Build history of the part. All positions in model axes, mm. A direction names the side the tool comes from. Round coordinates to 2 decimals unless told otherwise and drop trailing zeros. Write each loop counter-clockwise with the first axis right and the second up, starting at its lowest first coordinate (ties: lowest second). Pieces come first, ordered by that corner, then holes. Notation, with made-up numbers: M 9,79 L 37,79 A16 cw 37,110 Z; hole C 44.5,77 d9. An arc over 180 degrees is marked long. Write item = value, one per line.
Autodesk Fusion 360 part; units mm, degrees
sketch "Sketch1" plane through (0, 0, 0) normal (0, 1, 0) x (1, 0, 0)
  line L0 (0, 0) -> (88, 0)
  line L1 (88, 0) -> (88, 8.2)
  line L2 (88, 8.2) -> (0, 8.2)
  line L3 (0, 8.2) -> (0, 0)
  dimension "d1" = 88
  dimension "d2" = 8.2
extrude "Extrude1" add sketch "Sketch1" along normal blind 12.75
sketch "Sketch2" plane through (0, 12.75, 0) normal (0, 1, 0) x (-1, 0, 0)
  line L0 (0, -8.2) -> (0, 0)
  line L1 (0, 0) -> (-88, 0)
  line L2 (-88, 0) -> (-88, -8.2)
  line L3 (-88, -8.2) -> (0, -8.2)
  line L4 (0, 0) -> (-6.77, 0)
  line L5 (-6.77, 0) -> (-6.77, -8.2)
  line L6 (-6.77, -8.2) -> (0, -8.2)
  line L7 (0, -8.2) -> (0, 0)
  line L8 (-6.77, -8.2) -> (-13.54, -8.2)
  line L9 (-13.54, -8.2) -> (-13.54, 0)
  line L10 (-13.54, 0) -> (-6.77, 0)
  line L11 (-6.77, 0) -> (-6.77, -8.2)
  dimension "d5" = 6.77
  dimension "d6" = 6.77
extrude "Extrude2" cut sketch "Sketch2" against normal blind 6.5 contours L1 L3 L5 L8 L9 L10 L11
sketch "Sketch3" plane through (0, 12.75, 0) normal (0, 1, 0) x (-1, 0, 0)
  line L0 (-13.54, -8.2) -> (-13.54, 0)
  line L1 (-13.54, 0) -> (-88, 0)
  line L2 (-88, 0) -> (-88, -8.2)
  line L3 (-88, -8.2) -> (-13.54, -8.2)
  line L4 (-13.54, 0) -> (-20.31, 0)
  line L5 (-20.31, 0) -> (-20.31, -8.2)
  line L6 (-20.31, -8.2) -> (-13.54, -8.2)
  line L7 (-13.54, -8.2) -> (-13.54, 0)
  line L8 (-20.31, -8.2) -> (-27.08, -8.2)
  line L9 (-27.08, -8.2) -> (-27.08, 0)
  line L10 (-27.08, 0) -> (-20.31, 0)
  line L11 (-20.31, 0) -> (-20.31, -8.2)
  dimension "d9" = 6.77
  dimension "d10" = 6.77
extrude "Extrude3" cut sketch "Sketch3" against normal blind 6.5 contours L1 L3 L5 L8 L9 L10 L11
sketch "Sketch4" plane through (0, 12.75, 0) normal (0, 1, 0) x (-1, 0, 0)
  line L0 (-27.08, -8.2) -> (-27.08, 0)
  line L1 (-27.08, 0) -> (-88, 0)
  line L2 (-88, 0) -> (-88, -8.2)
  line L3 (-88, -8.2) -> (-27.08, -8.2)
  line L4 (-27.08, 0) -> (-33.85, 0)
  line L5 (-33.85, 0) -> (-33.85, -8.2)
  line L6 (-33.85, -8.2) -> (-27.08, -8.2)
  line L7 (-27.08, -8.2) -> (-27.08, 0)
  line L8 (-33.85, -8.2) -> (-40.62, -8.2)
  line L9 (-40.62, -8.2) -> (-40.62, 0)
  line L10 (-40.62, 0) -> (-33.85, 0)
  line L11 (-33.85, 0) -> (-33.85, -8.2)
  dimension "d13" = 6.77
  dimension "d14" = 6.77
extrude "Extrude4" cut sketch "Sketch4" against normal blind 6.5 contours L1 L3 L5 L8 L9 L10 L11
sketch "Sketch5" plane through (0, 12.75, 0) normal (0, 1, 0) x (-1, 0, 0)
  line L0 (-40.62, -8.2) -> (-40.62, 0)
  line L1 (-40.62, 0) -> (-88, 0)
  line L2 (-88, 0) -> (-88, -8.2)
  line L3 (-88, -8.2) -> (-40.62, -8.2)
  line L4 (-40.62, 0) -> (-47.39, 0)
  line L5 (-47.39, 0) -> (-47.39, -8.2)
  line L6 (-47.39, -8.2) -> (-40.62, -8.2)
  line L7 (-40.62, -8.2) -> (-40.62, 0)
  line L8 (-47.39, -8.2) -> (-54.16, -8.2)
  line L9 (-54.16, -8.2) -> (-54.16, 0)
  line L10 (-54.16, 0) -> (-47.39, 0)
  line L11 (-47.39, 0) -> (-47.39, -8.2)
  dimension "d17" = 6.77
  dimension "d18" = 6.77
extrude "Extrude5" cut sketch "Sketch5" against normal blind 6.5 contours L1 L3 L5 L8 L9 L10 L11
sketch "Sketch6" plane through (0, 12.75, 0) normal (0, 1, 0) x (-1, 0, 0)
  line L0 (-54.16, -8.2) -> (-54.16, 0)
  line L1 (-54.16, 0) -> (-88, 0)
  line L2 (-88, 0) -> (-88, -8.2)
  line L3 (-88, -8.2) -> (-54.16, -8.2)
  line L4 (-54.16, 0) -> (-60.93, 0)
  line L5 (-60.93, 0) -> (-60.93, -8.2)
  line L6 (-60.93, -8.2) -> (-54.16, -8.2)
  line L7 (-54.16, -8.2) -> (-54.16, 0)
  line L8 (-60.93, 0) -> (-67.7, 0)
  line L9 (-67.7, 0) -> (-67.7, -8.2)
  line L10 (-67.7, -8.2) -> (-60.93, -8.2)
  line L11 (-60.93, -8.2) -> (-60.93, 0)
  dimension "d21" = 6.77
  dimension "d22" = 6.77
extrude "Extrude6" cut sketch "Sketch6" against normal blind 6.5 contours L1 L3 L5 L8 L9 L10 L11
sketch "Sketch7" plane through (0, 12.75, 0) normal (0, 1, 0) x (-1, 0, 0)
  line L0 (-67.7, -8.2) -> (-67.7, 0)
  line L1 (-67.7, 0) -> (-88, 0)
  line L2 (-88, 0) -> (-88, -8.2)
  line L3 (-88, -8.2) -> (-67.7, -8.2)
  line L4 (-67.7, 0) -> (-74.47, 0)
  line L5 (-74.47, 0) -> (-74.47, -8.2)
  line L6 (-74.47, -8.2) -> (-67.7, -8.2)
  line L7 (-67.7, -8.2) -> (-67.7, 0)
  line L8 (-74.47, -8.2) -> (-81.24, -8.2)
  line L9 (-81.24, -8.2) -> (-81.24, 0)
  line L10 (-81.24, 0) -> (-74.47, 0)
  line L11 (-74.47, 0) -> (-74.47, -8.2)
  dimension "d25" = 6.77
  dimension "d26" = 6.77
extrude "Extrude7" cut sketch "Sketch7" against normal blind 6.5 contours L1 L3 L5 L8 L9 L10 L11
1. Flat gauge pin, fed straight in: pin 1 (3.5 mm diameter, centred on x = 51, z = -5, fed in from +Y). Where does the tip first touch, or does it go through?
Responses:
pin_1 = 6.25
2. Mould opens along X. For faces 3 (the face through (0, 6, -4)), 4 (the face through (85, 12.75, -4)), 5 (the face through (60.93, 10, -4)) say: pulls with the +X half, pulls with the -X half, needs draft (parallel to the pull), parting line crosses it, or undercut.
Responses:
face_3 = pulls with the -X half
face_4 = needs draft
face_5 = undercut
3. Band-saw the part on B-B (z = -7.25). List the corners of the cut face in (x, y).
Responses:
outline = M 0,0 L 88,0 L 88,12.75 L 81.24,12.75 L 81.24,6.25 L 74.47,6.25 L 74.47,12.75 L 67.7,12.75 L 67.7,6.25 L 60.93,6.25 L 60.93,12.75 L 54.16,12.75 L 54.16,6.25 L 47.39,6.25 L 47.39,12.75 L 40.62,12.75 L 40.62,6.25 L 33.85,6.25 L 33.85,12.75 L 27.08,12.75 L 27.08,6.25 L 20.31,6.25 L 20.31,12.75 L 13.54,12.75 L 13.54,6.25 L 6.77,6.25 L 6.77,12.75 L 0,12.75 Z
4. Band-saw the part on A-A (y = 10). List the corners of the cut face in (x, z), plus the area to 3 significant figures.
Responses:
outline = M 0,-8.2 L 6.77,-8.2 L 6.77,0 L 0,0 Z; M 13.54,-8.2 L 20.31,-8.2 L 20.31,0 L 13.54,0 Z; M 27.08,-8.2 L 33.85,-8.2 L 33.85,0 L 27.08,0 Z; M 40.62,-8.2 L 47.39,-8.2 L 47.39,0 L 40.62,0 Z; M 54.16,-8.2 L 60.93,-8.2 L 60.93,0 L 54.16,0 Z; M 67.7,-8.2 L 74.47,-8.2 L 74.47,0 L 67.7,0 Z; M 81.24,-8.2 L 88,-8.2 L 88,0 L 81.24,0 Z
area = 389 mm²
5. Band-saw the part on C-C (x = 52.5). List the corners of the cut face in (y, z).
Responses:
outline = M 0,-8.2 L 6.25,-8.2 L 6.25,0 L 0,0 Z
6. Probe probe 1 along Y at (x, z) = (62, -7.75). List the from-to ranges inside material, lowest first.
Responses:
probe_1 = 0 to 6.25
7. Tool access for faces 1 (the face through (43, 0, -4)), 2 (the face through (54.16, 10, -4)): list every direction of +Z, -Z, +X, -X, +Y, -Y with a clear straight run to the whole face (end or side of a thin tool).
Responses:
face_1 = +Z, -Z, +X, -X, -Y
face_2 = +Z, -Z, +Y
